```python
from build123d import *

# Parameters (mm, degrees)
BOSS_EXTRUDE1_DEPTH            = 76.2
SKETCH2_R                      = 12.7
CUT_EXTRUDE1_DEPTH             = 132.982271537
F_5_16_0_3125_DIAMETER_HOLE1_D = 7.9375
LPATTERN1_COUNT                = 2
LPATTERN1_PITCH                = 38.1
LPATTERN1_COUNT_DIR2           = 2
LPATTERN1_PITCH_DIR2           = 38.1


with BuildPart() as part:
    # Sketch1 → Boss-Extrude1 (new body)
    with BuildSketch(Plane(origin=(0, 0, 0), x_dir=(0, 0, -1), z_dir=(1, 0, 0))):
        Polygon((0, 0), (76.2, 0), (76.2, 76.2), (63.5, 76.2), (63.5, 12.7), (12.7, 12.7), (12.7, 76.2), (0, 76.2), align=None)
    extrude(amount=BOSS_EXTRUDE1_DEPTH)

    # Sketch2 → Cut-Extrude1 (cut, through all)
    with BuildSketch(Plane.XY):
        with Locations((38.1, 50.8)):
            Circle(SKETCH2_R)
    extrude(amount=-CUT_EXTRUDE1_DEPTH, mode=Mode.SUBTRACT)

    # 5/16 (0.3125) Diameter Hole1 (through all)
    with Locations(Plane(origin=(0, 12.7, 0), x_dir=(1, 0, 0), z_dir=(0, 1, 0))):
        with Locations((19.05, 19.05)):
            f_5_16_0_3125_diameter_hole1 = Hole(F_5_16_0_3125_DIAMETER_HOLE1_D / 2)

    # LPattern1: 5_16 _0.3125_ Diameter Hole1 2 × 2
    with Locations(*[(i * LPATTERN1_PITCH, 0, -j * LPATTERN1_PITCH_DIR2) for i in range(LPATTERN1_COUNT) for j in range(LPATTERN1_COUNT_DIR2) if (i, j) != (0, 0)]):
        add(f_5_16_0_3125_diameter_hole1, mode=Mode.SUBTRACT)


solid = part.part
```
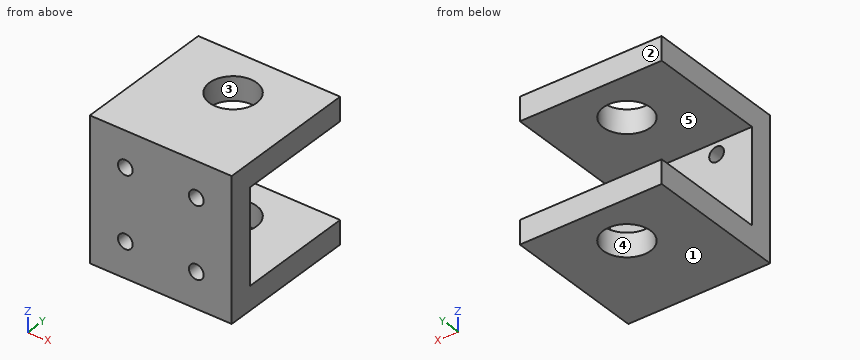
CAD build for the part. Positions are in the model's coordinates, mm. Face numbers are marked on the shaded views. A direction names the side the tool comes from. Round coordinates to 2 decimals unless told otherwise and drop trailing zeros. Order: outer loops, then holes, each group sorted by start corner. A loop starts at its lowest first (then second) coordinate and runs counter-clockwise, first axis right, second up.
Item 1: Tool access for the marked faces 4 and 5: list every direction of +Z, -Z, +X, -X, +Y, -Y with a clear straight run to the whole face (end or side of a thin tool).
Item 2: Mould opens along Y. For the marked faces 1, 2 and 3 say: pulls with the +Y half, pulls with the -Y half, needs draft (parallel to the pull), parting line crosses it, or undercut.
Item 3: Saw through at D-D on y = 21.5. Write the cut outline in (x, z), then the cut area to 3 significant figures.
Item 4: Saw through at A-A on x = 38.1. Write the cut outline in (y, z).
Item 5: Probe line 1 along X through (y, z) = (5.25, -19.05); line 2 along Z through (x, y) = (19, 3); line 3 along Z through (x, y) = (70.5, 67.5). List the from-to ranges inside material, lowest first.
Item 6: Pin check, flat tips, straight feed: pin 1 (10.5 mm diameter, centred on x = 19.05, z = -19.05, fed in from -Y); pin 2 (1 mm diameter, centred on x = 32, y = 41, fed in from -Z); pin 3 (6 mm diameter, centred on x = 51.5, z = -37.5, fed in from +Y). Stop position of each tip, or through.
Item 7: Saw through at C-C on y = 50.8. Write the cut outline in (x, z), then the cut area to 3 significant figures.
Item 8: Saw through at B-B on z = -19.05. Write the cut outline in (x, y), then the cut area to 3 significant figures.
Reported:
1. face 4: +Z, -Z
1. face 5: +X, -X, +Y
2. face 1: needs draft
2. face 2: pulls with the +Y half
2. face 3: undercut
3. outline: (0, -76.2) - (76.2, -76.2) - (76.2, -63.5) - (0, -63.5) - close; (0, -12.7) - (76.2, -12.7) - (76.2, 0) - (0, 0) - close
3. area: 1,940 mm2
4. outline: (0, -76.2) - (38.1, -76.2) - (38.1, -63.5) - (12.7, -63.5) - (12.7, -12.7) - (38.1, -12.7) - (38.1, 0) - (0, 0) - close; (63.5, -76.2) - (76.2, -76.2) - (76.2, -63.5) - (63.5, -63.5) - close; (63.5, -12.7) - (76.2, -12.7) - (76.2, 0) - (63.5, 0) - close
5. line 1: x = 0 to 15.08, 23.02 to 53.18, 61.12 to 76.2
5. line 2: z = -76.2 to -61.12, -53.18 to -23.02, -15.08 to 0
5. line 3: z = -76.2 to -63.5, -12.7 to 0
6. pin 1: stops at y = 0
6. pin 2: passes through
6. pin 3: stops at y = 12.7
7. outline: (0, -76.2) - (25.4, -76.2) - (25.4, -63.5) - (0, -63.5) - close; (0, -12.7) - (25.4, -12.7) - (25.4, 0) - (0, 0) - close; (50.8, -76.2) - (76.2, -76.2) - (76.2, -63.5) - (50.8, -63.5) - close; (50.8, -12.7) - (76.2, -12.7) - (76.2, 0) - (50.8, 0) - close
7. area: 1,290 mm2
8. outline: (0, 0) - (15.08, 0) - (15.08, 12.7) - (0, 12.7) - close; (23.02, 0) - (53.18, 0) - (53.18, 12.7) - (23.02, 12.7) - close; (61.12, 0) - (76.2, 0) - (76.2, 12.7) - (61.12, 12.7) - close
8. area: 766 mm2
